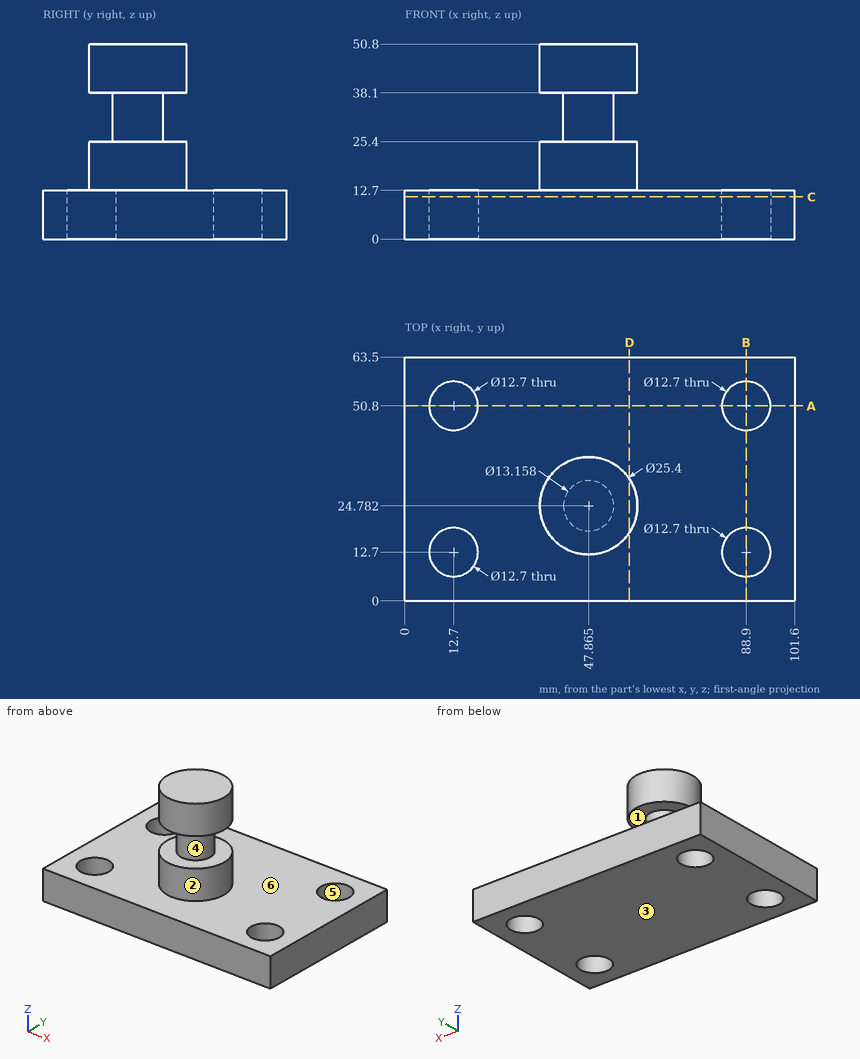
Geometry check sheet. Reference: drawing and pictorial views, mm from the part's lowest x, y, z. A direction names the side the tool comes from. Round coordinates to 2 decimals unless told otherwise and drop trailing zeros. Write each loop counter-clockwise with the first axis right and the second up, starting at its lowest first coordinate (ties: lowest second). Pieces come first, ordered by that corner, then holes. Notation, with made-up numbers: (-8, -26.75) -> (2, -26.75) arc R18 ccw to (2, -9.75) -> close; hole circle Ø5 at (72, -40). An arc over 180 degrees is marked (long way). Put each result on its own line as item: value.
1) Depth check by flat-ended pin: P1, Ø5, axis at y = 36, z = 24, coming from the +X side; P2, Ø5, axis at x = 26.5, y = 14, coming from the +Z side; P3, Ø12, axis at y = 30.5, z = 36.5, coming from the -X side (1 decimal). Enter the tip coordinate at first touch or a pass-through.
Recorded:
P1: stops at x = 57.1
P2: stops at z = 12.7
P3: stops at x = 35.2
2) Access from +Z, -Z, +X, -X, +Y, -Y to the whole of each face (thin tool, end or side, straight path). Record for the marked faces 1, 2 and 3.
Recorded:
face 1: none
face 2: +Z
face 3: -Z, +X, -X, +Y, -Y
3) Thickness scan on probe 1 along Y at (x, z) = (88.9, 4.5); probe 2 along X at (y, z) = (50, 7); probe 3 along Z at (x, y) = (6, 25). Record the ranges inside material, lowest first. Write a range as from..to.
Recorded:
probe 1: y = 0..6.35, 19.05..44.45, 57.15..63.5
probe 2: x = 0..6.4, 19..82.6, 95.2..101.6
probe 3: z = 0..12.7
4) Cross-section at C-C, the plane z = 11. Enter the section's corners in (x, y), plus the area to 4 significant figures.
Recorded:
outline: (0, 0) -> (101.6, 0) -> (101.6, 63.5) -> (0, 63.5) -> close; hole circle Ø12.7 at (12.7, 12.7); hole circle Ø12.7 at (12.7, 50.8); hole circle Ø12.7 at (88.9, 12.7); hole circle Ø12.7 at (88.9, 50.8)
area: 5,945 mm2
5) Cross-section at D-D, the plane x = 58.5. Enter the section's corners in (y, z) (1 decimal), plus the area to 3 significant figures.
Recorded:
outline: (0, 0) -> (63.5, 0) -> (63.5, 12.7) -> (31.7, 12.7) -> (31.7, 25.4) -> (17.8, 25.4) -> (17.8, 12.7) -> (0, 12.7) -> close; (17.8, 38.1) -> (31.7, 38.1) -> (31.7, 50.8) -> (17.8, 50.8) -> close
area: 1,160 mm2
6) Cross-section at B-B, the plane x = 88.9. Enter the section's corners in (y, z).
Recorded:
outline: (0, 0) -> (6.35, 0) -> (6.35, 12.7) -> (0, 12.7) -> close; (19.05, 0) -> (44.45, 0) -> (44.45, 12.7) -> (19.05, 12.7) -> close; (57.15, 0) -> (63.5, 0) -> (63.5, 12.7) -> (57.15, 12.7) -> close
7) Release check for a two-part mould opening along Z. For the marked faces 4, 5 and 6 record: pulls with the +Z half, pulls with the -Z half, needs draft (parallel to the pull), parting line crosses it, or undercut.
Recorded:
face 4: undercut
face 5: needs draft
face 6: pulls with the +Z half
8) Cross-section at A-A, the plane y = 50.8. Enter the section's corners in (x, z), plus the area to 3 significant figures.
Recorded:
outline: (0, 0) -> (6.35, 0) -> (6.35, 12.7) -> (0, 12.7) -> close; (19.05, 0) -> (82.55, 0) -> (82.55, 12.7) -> (19.05, 12.7) -> close; (95.25, 0) -> (101.6, 0) -> (101.6, 12.7) -> (95.25, 12.7) -> close
area: 968 mm2
